from build123d import *

# Parameters (mm, degrees)
SKETCH_1_W                  = 50
SKETCH_1_H                  = 48
EXTRUDE_1_DEPTH             = 15
HOLE_WIZARD_M5_1_AT_2_COUNT = 2
HOLE_WIZARD_M5_1_AT_2_PITCH = 35
HOLE_WIZARD_M5_1_AT_3_COUNT = 2
HOLE_WIZARD_M5_1_AT_3_PITCH = 49.497474683
HOLE_WIZARD_M5_1_AT_4_COUNT = 2
HOLE_WIZARD_M5_1_AT_4_PITCH = 35
FILLET_1_R                  = 1
EXTRUDE_2_DEPTH             = 100
SKETCH_11_3_W               = 21
SKETCH_11_3_H               = 11.5
SKETCH_11_3_R               = 3.3
SKETCH_11_3_W_2             = 12.5
SKETCH_11_3_H_2             = 21
EXTRUDE_3_DEPTH             = 2
SKETCH_12_W                 = 50
SKETCH_12_H                 = 15
CUT_EXTRUDE_1_DEPTH         = 135.272111773
FILLET_3_R                  = 0.5


with BuildPart() as part:
    # Sketch 1 → Extrude 1 (new body)
    with BuildSketch(Plane.XY):
        with Locations((25, -24)):
            Rectangle(SKETCH_1_W, SKETCH_1_H)
    extrude(amount=EXTRUDE_1_DEPTH)

    # Sketch 4 → Hole Wizard M5 _1 (revolve, cut)
    with BuildSketch(Plane(origin=(7.5, -6.5, 15), x_dir=(0, -1, 0), z_dir=(1, 0, 0))):
        Polygon((0, 0), (0, 15), (2.75, 15), (2.75, 6), (5, 6), (5, 0.025), (5.025, 0), align=None)
    hole_wizard_m5_1 = revolve(axis=Axis((7.5, -6.5, 21.35), (0, 0, -1)), mode=Mode.SUBTRACT)

    # Hole Wizard M5 _1 at 2: Hole Wizard M5 _1 ×2
    with Locations(*[(i * HOLE_WIZARD_M5_1_AT_2_PITCH, 0, 0) for i in range(1, HOLE_WIZARD_M5_1_AT_2_COUNT)]):
        add(hole_wizard_m5_1, mode=Mode.SUBTRACT)

    # Hole Wizard M5 _1 at 3: Hole Wizard M5 _1 ×2
    with Locations(*[Vector(0.7071067811865476, -0.7071067811865476, 0) * (i * HOLE_WIZARD_M5_1_AT_3_PITCH) for i in range(1, HOLE_WIZARD_M5_1_AT_3_COUNT)]):
        add(hole_wizard_m5_1, mode=Mode.SUBTRACT)

    # Hole Wizard M5 _1 at 4: Hole Wizard M5 _1 ×2
    with Locations(*[(0, -i * HOLE_WIZARD_M5_1_AT_4_PITCH, 0) for i in range(1, HOLE_WIZARD_M5_1_AT_4_COUNT)]):
        add(hole_wizard_m5_1, mode=Mode.SUBTRACT)

    # Fillet 1
    fillet_1_edges = [part.edges().sort_by_distance(p)[0] for p in [
        (0, 0, 7.5),
        (50, 0, 7.5),
        (50, -48, 7.5),
        (0, -48, 7.5),
    ]]
    fillet(fillet_1_edges, radius=FILLET_1_R)

    # Sketch 10 → Hole Wizard M8 _1 (revolve, cut)
    with BuildSketch(Plane(origin=(25, -24, 0), x_dir=(0, 1, 0), z_dir=(1, 0, 0))):
        Polygon((0, 0), (0, 15), (4.5, 15), (4.5, 10), (7.5, 10), (7.5, 0.025), (7.525, 0), align=None)
    revolve(axis=Axis((25, -24, -6.35), (0, 0, 1)), mode=Mode.SUBTRACT)

    # Sketch 11 → Extrude 2 (add)
    with BuildSketch(Plane.XY.offset(15)):
        Polygon((14.5, -11.5), (12.5, -11.5), (12.5, -13.5), (12.5, -24), (14.5, -24), (14.5, -13.5), (25, -13.5), (25, -11.5), align=None)
        Polygon((35.5, -11.5), (25, -11.5), (25, -13.5), (35.5, -13.5), (35.5, -24), (37.5, -24), (37.5, -13.5), (37.5, -11.5), (36.5, -11.5), align=None)
        Polygon((37.5, -24), (35.5, -24), (35.5, -34.5), (25, -34.5), (25, -36.5), (35.5, -36.5), (37.5, -36.5), (37.5, -34.5), align=None)
        Polygon((14.5, -24), (12.5, -24), (12.5, -34.5), (12.5, -36.5), (14.5, -36.5), (25, -36.5), (25, -34.5), (14.5, -34.5), align=None)
    extrude(amount=EXTRUDE_2_DEPTH)

    # Sketch 11_3 → Extrude 3 (add)
    # profile 1 of 4: a face of its own
    with BuildSketch(Plane.XY.offset(15)):
        with Locations((25, -5.75)):
            Rectangle(SKETCH_11_3_W, SKETCH_11_3_H)
        with Locations((25, -6.5)):
            Circle(SKETCH_11_3_R, mode=Mode.SUBTRACT)
    # profile 2 of 4: a face of its own
    with BuildSketch(Plane.XY.offset(15)):
        with Locations((6.25, -24)):
            Rectangle(SKETCH_11_3_W_2, SKETCH_11_3_H_2)
        with Locations((7.5, -24)):
            Circle(SKETCH_11_3_R, mode=Mode.SUBTRACT)
    # profile 3 of 4: a face of its own
    with BuildSketch(Plane.XY.offset(15)):
        with Locations((25, -42.25)):
            Rectangle(SKETCH_11_3_W, SKETCH_11_3_H)
        with Locations((25, -41.5)):
            Circle(SKETCH_11_3_R, mode=Mode.SUBTRACT)
    # profile 4 of 4: a face of its own
    with BuildSketch(Plane.XY.offset(15)):
        with Locations((43.75, -24)):
            Rectangle(SKETCH_11_3_W_2, SKETCH_11_3_H_2)
        with Locations((42.5, -24)):
            Circle(SKETCH_11_3_R, mode=Mode.SUBTRACT)
    extrude(amount=EXTRUDE_3_DEPTH)

    # Sketch 12 → Cut-Extrude 1 (cut, through all)
    with BuildSketch(Plane.XZ.offset(48)):
        with Locations((25, 7.5)):
            Rectangle(SKETCH_12_W, SKETCH_12_H)
    extrude(amount=-CUT_EXTRUDE_1_DEPTH, mode=Mode.SUBTRACT)

    # Fillet 3
    fillet_3_edges = [part.edges().sort_by_distance(p)[0] for p in [
        (0, -34.5, 16),
        (0, -13.5, 16),
        (35.5, -48, 16),
        (14.5, -48, 16),
        (50, -13.5, 16),
        (50, -34.5, 16),
        (14.5, 0, 16),
        (35.5, 0, 16),
    ]]
    fillet(fillet_3_edges, radius=FILLET_3_R)


solid = part.part
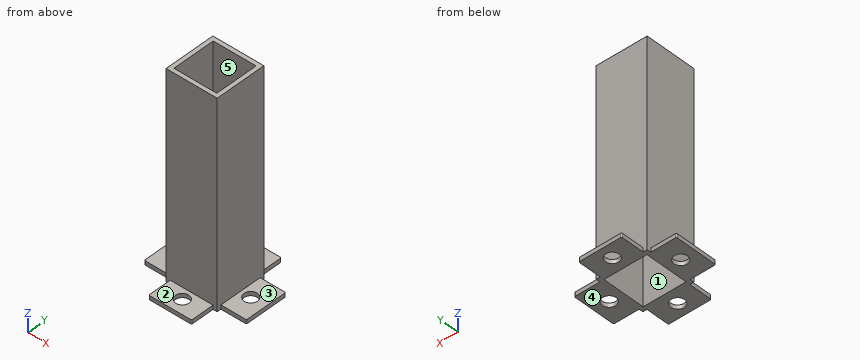
Part model, mm, in its own coordinate system. Face numbers are marked on the shaded views. A direction names the side the tool comes from. Give positions to 0.01 mm unless a question says otherwise; leave off trailing zeros. Loops run counter-clockwise (first coordinate to the right, second up) from the corner with the lowest first, then second, coordinate; pieces in that order, holes last.
(1) 3-axis set-ups, long thin cutter, end or side, ignore diameter. For the marked faces 3, 4 and 5: which of +Z, -Z, +X, -X, +Y, -Y reach the whole face in a straight line?
Return value:
face 3: +Z, +X, +Y, -Y
face 4: -Z, +X, -X, +Y, -Y
face 5: +Z, -Z
(2) Band-saw the part on B-B (y = -24). Write the cut outline in (x, z), and give its area (3 significant figures).
Return value:
outline: (0, 15) - (4.2, 15) - (4.2, 17) - (0, 17) - close; (10.8, 15) - (14.5, 15) - (14.5, 115) - (12.5, 115) - (12.5, 17) - (10.8, 17) - close; (35.5, 15) - (39.2, 15) - (39.2, 17) - (37.5, 17) - (37.5, 115) - (35.5, 115) - close; (45.8, 15) - (50, 15) - (50, 17) - (45.8, 17) - close
area: 424 mm2
(3) Drill centre lines: line 1 along Y through (x, z) = (25, 16.05); line 2 along Y through (x, z) = (34, 21.5); line 3 along X through (y, z) = (-14, 25.5). Where is each one in solid material? Low to high.
Return value:
line 1: y = -48 to -44.8, -38.2 to -34.5, -13.5 to -9.8, -3.2 to 0
line 2: y = -36.5 to -34.5, -13.5 to -11.5
line 3: x = 12.5 to 14.5, 35.5 to 37.5
(4) Pull direction Y, two halves, no side cores. Call the marked faces 1 and 2: pulls with the +Y half, pulls with the -Y half, needs draft (parallel to the pull), parting line crosses it, or undercut.
Return value:
face 1: undercut
face 2: needs draft
(5) Band-saw the part on A-A (x = 7.5). Write the cut outline in (y, z), and give its area (3 significant figures).
Return value:
outline: (-34.5, 15) - (-27.3, 15) - (-27.3, 17) - (-34.5, 17) - close; (-20.7, 15) - (-13.5, 15) - (-13.5, 17) - (-20.7, 17) - close
area: 28.8 mm2
(6) Band-saw the part on C-C (x = 25). Write the cut outline in (y, z), and give its area (3 significant figures).
Return value:
outline: (-48, 15) - (-44.8, 15) - (-44.8, 17) - (-48, 17) - close; (-38.2, 15) - (-34.5, 15) - (-34.5, 115) - (-36.5, 115) - (-36.5, 17) - (-38.2, 17) - close; (-13.5, 15) - (-9.8, 15) - (-9.8, 17) - (-11.5, 17) - (-11.5, 115) - (-13.5, 115) - close; (-3.2, 15) - (0, 15) - (0, 17) - (-3.2, 17) - close
area: 420 mm2
(7) Pin check, flat tips, straight feed: pin 1 (3.5 mm diameter, centred on x = 21.5, y = -3, fed in from +Z); pin 2 (1 mm diameter, centred on y = -6, z = 16.5, fed in from +X); pin 3 (0.6 mm diameter, centred on x = 41, z = 16.5, fed in from +Y). Stop position of each tip, or through.
Return value:
pin 1: stops at z = 17
pin 2: stops at x = 35.5
pin 3: stops at y = -13.5
(8) Band-saw the part on D-D (z = 50.5). Write the cut outline in (x, y).
Return value:
outline: (12.5, -36.5) - (37.5, -36.5) - (37.5, -11.5) - (12.5, -11.5) - close; hole (14.5, -34.5) - (35.5, -34.5) - (35.5, -13.5) - (14.5, -13.5) - close
